Source: three-view drawing plus pictorial views. Frame: mm from the lowest corner of the part. A direction names the side the tool comes from. Round coordinates to 2 decimals unless told otherwise and drop trailing zeros. Loops run counter-clockwise (first coordinate to the right, second up) from the corner with the lowest first, then second, coordinate; pieces in that order, holes last. Notation, with made-up numbers: M 50,-27 L 80,-27 A24 cw 80,-1 Z; hole C 16.25,89.25 d9. An arc over 180 degrees is marked long. Return JSON: item names as keys, results as strings. Group by question number.
1) Contact query for flat-ended pins moving along their axis: P1, Ø1, axis at x = 23, y = 23.5, coming from the -Z side; P2, Ø1.5, axis at x = 35.5, z = 9, coming from the +Y side; P3, Ø6, axis at x = 24.5, y = 22, coming from the -Z side; P4, Ø4.5, axis at x = 62.23, z = 15.875, coming from the -Y side. Output: stop coordinate, or through.
2) Section C-C (y = 5). Output: boundary loops of the cut face in (x, z), plus the area to 3 significant figures.
3) Access query for the marked faces 1 and 2. Directions: +Z, -Z, +X, -X, +Y, -Y. A direction counts if a zero-diameter tool reaches every point of the face in a straight line with its end or side. Return the directions, or none.
4) Material intervals for line 1 (X direction, y = 18, z = 16); line 2 (X direction, y = 25, z = 26.5); line 3 (Z direction, x = 62.23, y = 22.25), sorted ascending. Write a range as from..to.
5) Section A-A (x = 39). Output: boundary loops of the cut face in (y, z) (3 decimals), plus the area to 3 significant figures.
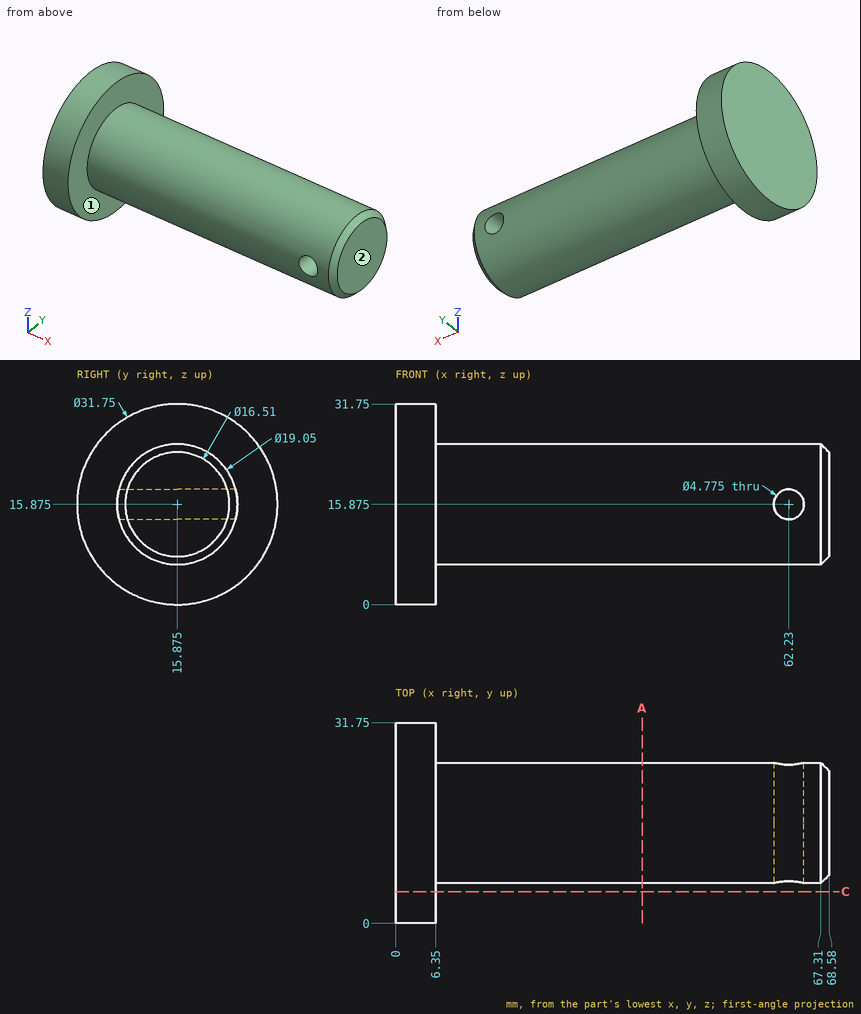
Returned:
{
 "1": {"P1": "stops at z = 9.55", "P2": "stops at y = 23.17", "P3": "stops at z = 6.88", "P4": "passes through"},
 "2": {"outline": "M 0,4.31 L 6.35,4.31 L 6.35,27.44 L 0,27.44 Z", "area": "147 mm^2"},
 "3": {"face 1": "+X", "face 2": "+Z, -Z, +X, +Y, -Y"},
 "4": {"line 1": "x = 0..59.85, 64.61..68.58", "line 2": "x = 0..6.35", "line 3": "z = 8.8..13.49, 18.26..22.95"},
 "5": {"outline": "C 15.875,15.875 d19.05", "area": "285 mm^2"}
}
